Build history of the part. All positions in model axes, mm. Face numbers are marked on the shaded views. A direction names the side the tool comes from. Round coordinates to 2 decimals unless told otherwise and drop trailing zeros. Order: outer loops, then holes, each group sorted by start corner. A loop starts at its lowest first (then second) coordinate and runs counter-clockwise, first axis right, second up. Notation, with made-up numbers: (-30, 30.5) - (15, 30.5) arc R20 ccw to (15, 43.5) - close; hole circle Ø3 at (9.5, -5.5). An arc over 180 degrees is marked (long way). Write each question's results on one line, items separated by ' | '. Start each with the question number.
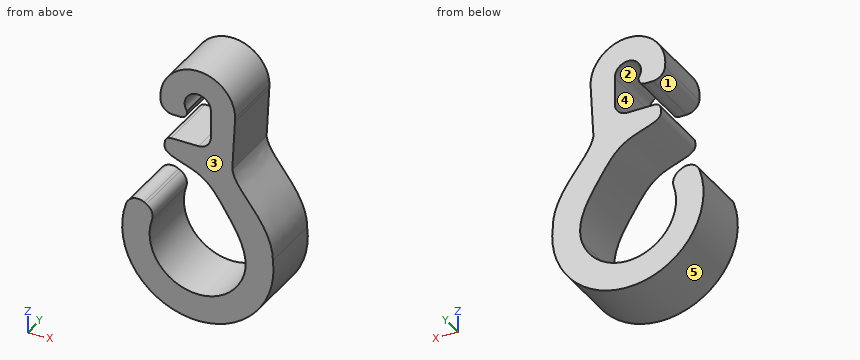
```python
from build123d import *

# Parameters (mm, degrees)
F1_DEPTH = 10
F2_R     = 1
F3_R     = 2


# Not quite as in the source:
# - two fillets or chamfers of one size are made in one step
# - a feature names something its author has since deleted; it is built from what else it names


with BuildPart() as f1:
    # F0 (on Front) → F1 (new body)
    with BuildSketch(Plane.XZ):
        with BuildLine():
            ThreePointArc((-1.7285399627, -1.1925391387), (-0.6245262518, 2.0049855263), (2.1, 0))
            Line((2.1, 0), (2.1, -6.4722087772))
            Line((2.1, -6.4722087772), (-1.7285399627, -6.4722087772))
            Line((-1.7285399627, -6.4722087772), (-5.1270676777, -6.4722087772))
            add(Edge.make_bspline(
                [(-5.1270676777, -6.4722087772), (-5.2022797508, -7.1671189286), (-6.0866195882, -9.4345123751), (1.027351741, -10.4770430063), (4.526556097, -16.11453384), (8.4301587847, -22.1647756383), (7.4084669429, -25.7151645559)],
                knots=[0, 0, 0, 0, 0.1536701078, 0.4002962667, 0.6726958228, 1, 1, 1, 1], degree=3))
            ThreePointArc((7.4084669429, -25.7151645559), (-3.085024735, -30.5342112997), (-6.6922515438, -19.5649590981))
            Line((-6.6922515438, -19.5649590981), (-10.5016801666, -17.3630853307))
            ThreePointArc((-10.5016801666, -17.3630853307), (-2.3664943525, -35.3449464187), (12.0481319901, -21.8635843278))
            add(Edge.make_bspline(
                [(5.535574435, -8.7558477202), (5.8434484166, -10.2656725536), (7.9936891439, -13.1024488577), (12.074048333, -18.3231807373), (12.0481319901, -21.8635843278)],
                knots=[0, 0, 0, 0, 0.4156437378, 1, 1, 1, 1], degree=3))
            Line((5.535574435, -8.7558477202), (5.9663335796, -0.6347153824))
            Line((5.9663335796, -0.6347153824), (6, 0))
            ThreePointArc((6, 0), (-1.2645054368, 5.8652387846), (-5.4670086667, -2.4722087772))
            Line((-5.4670086667, -2.4722087772), (-1.7285399627, -2.4722087772))
            Line((-1.7285399627, -2.4722087772), (-1.7285399627, -1.1925391387))
        make_face()
    extrude(amount=F1_DEPTH)

    # F2
    f2_edges = [f1.edges().sort_by_distance(p)[0] for p in [
        (-1.72854, -5, -2.472209),
        (-5.127068, -5, -6.472209),
    ]]
    fillet(f2_edges, radius=F2_R)

    # F3
    f3_edges = [f1.edges().sort_by_distance(p)[0] for p in [
        (-10.50168, -5, -17.363085),
        (-6.692252, -5, -19.564959),
        (-5.467009, -5, -2.472209),
        (2.1, -5, -6.472209),
    ]]
    fillet(f3_edges, radius=F3_R)


solid = f1.part
```
1. Mould opens along Z. For the marked faces 3, 4 and 5 say: pulls with the +Z half, pulls with the -Z half, needs draft (parallel to the pull), parting line crosses it, or undercut.
2. Cut at A-A (z = -3.5). List the corners of the cut face in (x, y), plus the area to 3 significant figures.
3. 3-axis set-ups, long thin cutter, end or side, ignore diameter. For the marked faces 1 and 2: which of +Z, -Z, +X, -X, +Y, -Y reach the whole face in a straight line?
4. Wall check: line 1 (Z direction, x = 0, y = -7.25); line 2 (Z direction, x = -1, y = -8.5); line 3 (X direction, y = -1, z = -25.5) (1 decimal). Give the ranges that are in metal, low to high. Write a range as from..to.
5. Flat gauge pins, fed straight in: pin 1 Ø5 at (y, z) = (-3.5, -1.5) entering from -X; pin 2 Ø2 at (x, y) = (-8, -5) entering from -Z; pin 3 Ø1.3 at (x, y) = (-2.5, -6.5) entering from +Z. Where does each tip first touch, or does it go through?
A:
1) face 3: needs draft | face 4: undercut | face 5: parting line crosses it
2) outline: (2.1, -10) - (5.81, -10) - (5.81, 0) - (2.1, 0) - close | area: 37.1 mm^2
3) face 1: -X, +Y, -Y | face 2: +Y, -Y
4) line 1: z = -35.58..-31.18, -11.04..-6.47, 2.1..6 | line 2: z = -35.54..-31.11, -10.58..-6.47, 1.85..5.92 | line 3: x = -12..-7.5, 7.5..12
5) pin 1: stops at x = -6 | pin 2: stops at z = -33.35 | pin 3: stops at z = 5.71
